```python
from build123d import *

# Parameters (mm, degrees)
F0_W     = 660.4
F0_H     = 304.8
F1_DEPTH = 6.35
F2_W     = 50.8
F2_H     = 50.8
F3_DEPTH = 6.35
F4_W     = 50.8
F4_H     = 6.35
F5_W     = 50.8
F5_H     = 6.35
F6_W     = 50.8
F6_H     = 6.35
F7_DEPTH = 44.45
F8_W     = 101.6
F8_H     = 50.8
F9_DEPTH = 9.525


with BuildPart() as f1:
    # F0 (on Front) → F1 (new body)
    with BuildSketch(Plane.XZ):
        Rectangle(F0_W, F0_H)
    extrude(amount=F1_DEPTH)

    # F2 (on face) → F3 (join)
    with BuildSketch(Plane.XZ.offset(6.35)):
        with Locations((254, -127)):
            Rectangle(F2_W, F2_H)
        with Locations((0, -127)):
            Rectangle(F2_W, F2_H)
        with Locations((-177.8, -127)):
            Rectangle(F2_W, F2_H)
    extrude(amount=F3_DEPTH)

    # F4 (on face) + F5 (on face) + F6 (on face) → F7 (join)
    with BuildSketch(Plane.XZ.offset(12.7)):
        with Locations((-177.8, -149.225)):
            Rectangle(F4_W, F4_H)
    with BuildSketch(Plane.XZ.offset(12.7)):
        with Locations((0, -149.225)):
            Rectangle(F5_W, F5_H)
    with BuildSketch(Plane.XZ.offset(12.7)):
        with Locations((254, -149.225)):
            Rectangle(F6_W, F6_H)
    extrude(amount=F7_DEPTH)

    # F8 (on face) → F9 (join)
    with BuildSketch(Plane(origin=(0, 0, 0), x_dir=(-1, 0, 0), z_dir=(0, 1, 0))):
        with Locations((-381, 101.6)):
            Rectangle(F8_W, F8_H)
        with Locations((-279.4, 101.6)):
            Rectangle(F8_W, F8_H)
    extrude(amount=F9_DEPTH)


solid = f1.part
```
Here's how the part is built. I have some questions about the finished solid (model axes, mm). A direction names the side the tool comes from. Coordinates: 2 decimals unless noted, no trailing zeros. Loops run counter-clockwise (first coordinate to the right, second up) from the corner with the lowest first, then second, coordinate; pieces in that order, holes last. Notation, with made-up numbers: M 45,-15 L 85,-15 A21 cw 85,12 Z; hole C 49.25,7.5 d2. An arc over 180 degrees is marked long. One line per item, written item: value.
1. Will these pins go through, and if not, where does the flat tip stop? pin 1 Ø22 at (x, y) = (-167, -31) entering from +Z; pin 2 Ø5 at (x, y) = (-10, -11) entering from +Z; pin 3 Ø1.9 at (y, z) = (-3, 49) entering from +X.
Geometry says:
pin 1: stops at z = -146.05
pin 2: stops at z = -101.6
pin 3: stops at x = 330.2
2. Imagine slicing it at A-A (y = -43). List the corners of the cut face in (x, z) for me.
Geometry says:
outline: M -203.2,-152.4 L -152.4,-152.4 L -152.4,-146.05 L -203.2,-146.05 Z; M -25.4,-152.4 L 25.4,-152.4 L 25.4,-146.05 L -25.4,-146.05 Z; M 228.6,-152.4 L 279.4,-152.4 L 279.4,-146.05 L 228.6,-146.05 Z
3. Imagine slicing it at D-D (z = 28). List the corners of the cut face in (x, y) for me.
Geometry says:
outline: M -330.2,-6.35 L 330.2,-6.35 L 330.2,0 L -330.2,0 Z
4. Imagine slicing it at C-C (x = 384). List the corners of the cut face in (y, z) for me (3 decimals).
Geometry says:
outline: M 0,76.2 L 9.525,76.2 L 9.525,127 L 0,127 Z
5. On a 3-axis mill with a long thin cutter (end or side, diameter ignored), from which of +Z, -Z, +X, -X, +Y, -Y can I reach the whole of each face in a straight line? I mean faces 1 (the flat face through (25.4, -20, -148)), 2 (the flat face through (254, -35, -146.05)), 3 (the flat face through (279.4, -20, -148)). Say none if no direction works.
Geometry says:
face 1: +Z, -Z, -Y
face 2: +Z, +X, -X, -Y
face 3: +Z, -Z, +X, -Y
6. Please list where these lines run through material, in increasing order: probe 1 along X at (y, z) = (-7, -140); probe 2 along Y at (x, z) = (-163, -61.5); probe 3 along Y at (x, z) = (383, 101.5) (3 decimals).
Geometry says:
probe 1: x = -203.2 to -152.4, -25.4 to 25.4, 228.6 to 279.4
probe 2: y = -6.35 to 0
probe 3: y = 0 to 9.525
7. Imagine slicing it at B-B (z = -110.5). List the corners of the cut face in (x, y) for me.
Geometry says:
outline: M -330.2,-6.35 L -203.2,-6.35 L -203.2,-12.7 L -152.4,-12.7 L -152.4,-6.35 L -25.4,-6.35 L -25.4,-12.7 L 25.4,-12.7 L 25.4,-6.35 L 228.6,-6.35 L 228.6,-12.7 L 279.4,-12.7 L 279.4,-6.35 L 330.2,-6.35 L 330.2,0 L -330.2,0 Z
